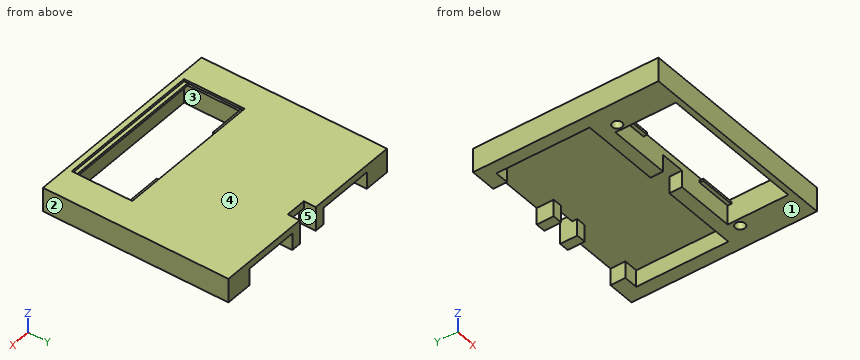
```python
from build123d import *

# Parameters (mm, degrees)
SKETCH1_W           = 215.166666666
SKETCH1_H           = 194.666666667
BOSS_EXTRUDE1_DEPTH = 25.4
SKETCH2_R           = 5.08
CUT_EXTRUDE1_DEPTH  = 17.78
SKETCH3_W           = 152.4
SKETCH3_H           = 63.5
CUT_EXTRUDE2_DEPTH  = 26.4
SKETCH4_W           = 21.718207711
SKETCH4_H           = 12.612953238
CUT_EXTRUDE3_DEPTH  = 26.4
SKETCH6_W           = 38.1
SKETCH6_H           = 2.54
SKETCH6_W_2         = 38.074968348
BOSS_EXTRUDE2_DEPTH = 3.81
SKETCH8_W           = 152.4
SKETCH8_H           = 2.54
BOSS_EXTRUDE3_DEPTH = 3.81
SKETCH9_W           = 2.54
SKETCH9_H           = 55.88
CUT_EXTRUDE8_DEPTH  = 3.81
SKETCH10_W          = 10.102446857
SKETCH10_H          = 17.859023659
SKETCH10_W_2        = 10.26192437
BOSS_EXTRUDE4_DEPTH = 17.78


with BuildPart() as part:
    # Sketch1 → Boss-Extrude1 (new body)
    with BuildSketch(Plane.XY):
        with Locations((78, 82.448428597)):
            Rectangle(SKETCH1_W, SKETCH1_H)
    extrude(amount=BOSS_EXTRUDE1_DEPTH)

    # Sketch2 → Cut-Extrude1 (cut)
    with BuildSketch(Plane(origin=(0, 0, 0), x_dir=(-1, 0, 0), z_dir=(0, 0, -1))):
        with Locations((5.416666667, 47.03176193)):
            Circle(SKETCH2_R)
        with Locations((-161.416666667, 47.03176193)):
            Circle(SKETCH2_R)
        Polygon((2.114639597, 179.78176193), (-157.022787609, 179.78176193), (-157.022787609, 164.200846175), (-171.765480067, 164.200846175), (-171.765480067, 67.571945264), (-148.766666667, 67.571945264), (-91.83014353, 67.571945264), (-91.83014353, 31.6046473), (-66.159852528, 31.6046473), (-66.159852528, 67.571945264), (-7.233333333, 67.387956716), (16.581678434, 67.387956716), (16.581678434, 165.292698163), (2.114639597, 165.292698163), align=None)
    extrude(amount=-CUT_EXTRUDE1_DEPTH, mode=Mode.SUBTRACT)

    # Sketch3 → Cut-Extrude2 (cut, through all)
    with BuildSketch(Plane(origin=(0, 0, 0), x_dir=(-1, 0, 0), z_dir=(0, 0, -1))):
        with Locations((-77.714845761, 22.583067422)):
            Rectangle(SKETCH3_W, SKETCH3_H)
    extrude(amount=-CUT_EXTRUDE2_DEPTH, mode=Mode.SUBTRACT)

    # Sketch4 → Cut-Extrude3 (cut, through all)
    with BuildSketch(Plane(origin=(0, 0, 0), x_dir=(-1, 0, 0), z_dir=(0, 0, -1))):
        with Locations((-77.933490884, 173.475285311)):
            Rectangle(SKETCH4_W, SKETCH4_H)
    extrude(amount=-CUT_EXTRUDE3_DEPTH, mode=Mode.SUBTRACT)

    # Sketch6 → Boss-Extrude2 (add)
    with BuildSketch(Plane.XZ.offset(-54.333067422)):
        with Locations((20.564845761, 21.59)):
            Rectangle(SKETCH6_W, SKETCH6_H)
        with Locations((134.877361587, 21.59)):
            Rectangle(SKETCH6_W_2, SKETCH6_H)
    extrude(amount=BOSS_EXTRUDE2_DEPTH)

    # Sketch8 → Boss-Extrude3 (add)
    with BuildSketch(Plane(origin=(0, -9.166932578, 0), x_dir=(1, 0, 0), z_dir=(0, 1, 0))):
        with Locations((77.714845761, -21.59)):
            Rectangle(SKETCH8_W, SKETCH8_H)
    extrude(amount=BOSS_EXTRUDE3_DEPTH)

    # Sketch9 → Cut-Extrude8 (cut)
    with BuildSketch(Plane(origin=(1.514845761, 0, 0), x_dir=(0, 0, -1), z_dir=(1, 0, 0))):
        with Locations((-21.59, 22.583067422)):
            Rectangle(SKETCH9_W, SKETCH9_H)
    extrude(amount=-CUT_EXTRUDE8_DEPTH, mode=Mode.SUBTRACT)

    # Sketch10 → Boss-Extrude4 (add)
    with BuildSketch(Plane(origin=(0, 0, 17.78), x_dir=(-1, 0, 0), z_dir=(0, 0, -1))):
        with Locations((-93.843818168, 170.852250101)):
            Rectangle(SKETCH10_W, SKETCH10_H)
        with Locations((-61.943424843, 170.852250101)):
            Rectangle(SKETCH10_W_2, SKETCH10_H)
    extrude(amount=BOSS_EXTRUDE4_DEPTH)


solid = part.part
```
Design review of the part built by this model. Coordinates are the model's own, in mm. Face numbers are marked on the shaded views. A direction names the side the tool comes from. Give positions to 0.01 mm unless a question says otherwise; leave off trailing zeros. Loops run counter-clockwise (first coordinate to the right, second up) from the corner with the lowest first, then second, coordinate; pieces in that order, holes last. Notation, with made-up numbers: (-38, 22) -> (-15, 22) arc R30 ccw to (-15, 60) -> close; hole circle Ø9 at (20.5, -19.5). An arc over 180 degrees is marked (long way). One line per item, written item: value.
Q1. For L1, parallel to X at y = 23, z = 15; L2, parallel to Y at x = 51.5, z = 3.5; L3, parallel to X at y = 167.5, z = 7, list the stretches that pass through material, from the lowest coordinate up.
Numbers:
L1: x = -29.58 to 1.51, 153.91 to 185.58
L2: y = -14.88 to -9.17, 54.33 to 67.53
L3: x = -29.58 to -2.11, 56.81 to 67.07, 88.79 to 98.9, 157.02 to 185.58
Q2. We need section D-D on y = 116. Give the boundary of the cut face in (x, z), and give its area (3 significant figures).
Numbers:
outline: (-29.58, 0) -> (-16.58, 0) -> (-16.58, 17.78) -> (171.77, 17.78) -> (171.77, 0) -> (185.58, 0) -> (185.58, 25.4) -> (-29.58, 25.4) -> close
area: 2,120 mm^2
Q3. Machinability: for the marked faces 4 and 5, which of the approach directions +Z, -Z, +X, -X, +Y, -Y give a long, thin tool a straight path to every point of the face, cutting with its end or side? Answer none if there is none.
Numbers:
face 4: +Z, +X, -X, +Y, -Y
face 5: -Z, +Y
Q4. We need section C-C on y = 9. Give the boundary of the cut face in (x, z).
Numbers:
outline: (-29.58, 0) -> (1.51, 0) -> (1.51, 20.32) -> (-2.3, 20.32) -> (-2.3, 22.86) -> (1.51, 22.86) -> (1.51, 25.4) -> (-29.58, 25.4) -> close; (153.91, 0) -> (185.58, 0) -> (185.58, 25.4) -> (153.91, 25.4) -> close
Q5. Draft analysis for pull direction X (two halves, no side actions). For the marked faces 1, 2 and 3, state which applies: pulls with the +X half, pulls with the -X half, needs draft (parallel to the pull), parting line crosses it, or undercut.
Numbers:
face 1: needs draft
face 2: pulls with the +X half
face 3: undercut
Q6. We need section A-A on z = 9.25. Give the number of separate pieces and of enclosed holes in the cut face, and give its area (3 significant figures).
Numbers:
separate pieces: 3
enclosed holes: 2
area: 11,400 mm^2
Q7. We need section B-B on x = 134. Give the boundary of the cut face in (y, z), and give its area (3 significant figures).
Numbers:
outline: (-14.88, 0) -> (-9.17, 0) -> (-9.17, 20.32) -> (-5.36, 20.32) -> (-5.36, 22.86) -> (-9.17, 22.86) -> (-9.17, 25.4) -> (-14.88, 25.4) -> close; (50.52, 20.32) -> (54.33, 20.32) -> (54.33, 0) -> (67.57, 0) -> (67.57, 17.78) -> (179.78, 17.78) -> (179.78, 25.4) -> (54.33, 25.4) -> (54.33, 22.86) -> (50.52, 22.86) -> close
area: 1,360 mm^2
Q8. For pin 1 Ø5 at (x, y) = (115, 85) entering from -Z; pin 2 Ø1 at (x, z) = (111.5, 13.5) entering from +Y; pin 3 Ø3 at (x, y) = (143, 51.5) entering from +Z; pin 4 Ø8 at (x, y) = (161.5, 49) entering from -Z, all flat-tipped, find the tip position at first contact; note any pin that passes through.
Numbers:
pin 1: stops at z = 17.78
pin 2: stops at y = 67.57
pin 3: stops at z = 22.86
pin 4: stops at z = 0
